Work out the finished part from the listing and answer in its coordinate system (mm). Face numbers are marked on the shaded views. A direction names the side the tool comes from. Round coordinates to 2 decimals unless told otherwise and drop trailing zeros. Order: outer loops, then holes, each group sorted by start corner. A loop starts at its lowest first (then second) coordinate and runs counter-clockwise, first axis right, second up. Notation, with made-up numbers: (-5, 21.5) - (29, 21.5) arc R19 cw to (29, 46.5) - close; hole circle Ø9 at (77, 37.5). An arc over 180 degrees is marked (long way). Use one line per item in the form item = value. Start each with the question number.
Q1. Given P1, Ø1, axis at x = 3, y = -2.5, coming from the -Z side; P2, Ø1.1, axis at y = 1, z = -48, coming from the -X side; P3, Ø1.5, axis at x = 4.5, z = -41.5, coming from the -Y side, each flat-ended and moving along its own axis, determine where each tip first touches the part or whether it passes through.
Q2. The part is cut by section A-A on z = -36.5. Determine the outline of the cut face in (x, y), plus the area to 3 significant figures.
Q3. Find the intervals of material crossed by line 1 (Y direction, x = 3.25, z = -34); line 2 (Z direction, x = 4.25, y = 2); line 3 (Y direction, x = 2, z = -36), in increasing order. Write a range as [from, to].
Q4. Which of the six approach directions +Z, -Z, +X, -X, +Y, -Y give full straight-line access (tool end or side, diameter ignored) to the marked faces 1 and 2?
Q5. The part is cut by section B-B on z = -46. Determine the outline of the cut face in (x, y).
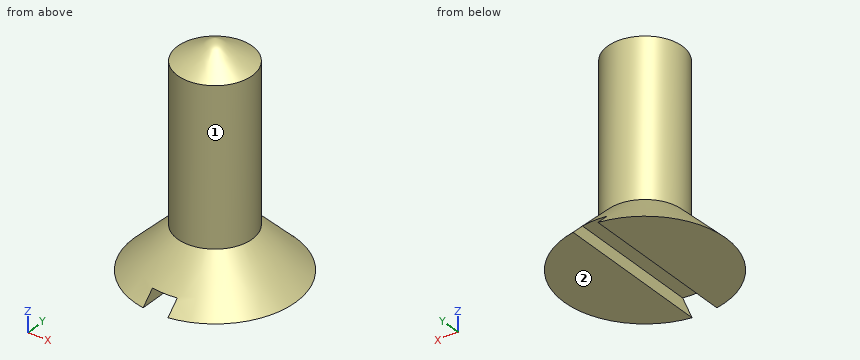
from build123d import *

# Parameters (mm, degrees)
CUT_EXTRUDE1_DEPTH      = 50.614070771
CUT_EXTRUDE1_DEPTH_BACK = 12
SKETCH2_W               = 2
SKETCH2_H               = 1


with BuildPart() as part:
    # Sketch1 → Revolve1 (revolve)
    with BuildSketch(Plane(origin=(0, 0, 0), x_dir=(1, 0, 0), z_dir=(0, 1, 0)), mode=Mode.PRIVATE) as revolve1_sk:
        Polygon((9.697241479, 48.221048581), (6.197241479, 44.721048581), (6.197241479, 32.221048581), (3.197241479, 30.488997773), (3.197241479, 48.221048581), align=None)
    revolve(revolve1_sk.sketch.rotate(Axis((3.197241479, 0, -48.221048581), (0, 0, 1)), 180), axis=Axis((3.197241479, 0, -48.221048581), (0, 0, 1)))

    # Sketch2 → Cut-Extrude1 (cut, two sides: drawn at the far end of the back side and taken through both)
    with BuildSketch(Plane(origin=(0, 0, 0), x_dir=(1, 0, 0), z_dir=(0, 1, 0)).offset(-CUT_EXTRUDE1_DEPTH_BACK)):
        with Locations((3.197241479, 47.721048581)):
            Rectangle(SKETCH2_W, SKETCH2_H)
    extrude(amount=CUT_EXTRUDE1_DEPTH + CUT_EXTRUDE1_DEPTH_BACK, mode=Mode.SUBTRACT)


solid = part.part
Found:
q1.P1 = -47.22
q1.P2 = -3.28
q1.P3 = -2.95
q2.outline = circle Ø6 at (3.2, 0)
q2.area = 28.3 mm²
q3.line_1 = [-3, 3]
q3.line_2 = [-48.22, -31.79]
q3.line_3 = [-2.75, 2.75]
q4.face_1 = +Z
q4.face_2 = -Z, +X, -X, +Y, -Y
q5.outline = circle Ø8.56 at (3.2, 0)
